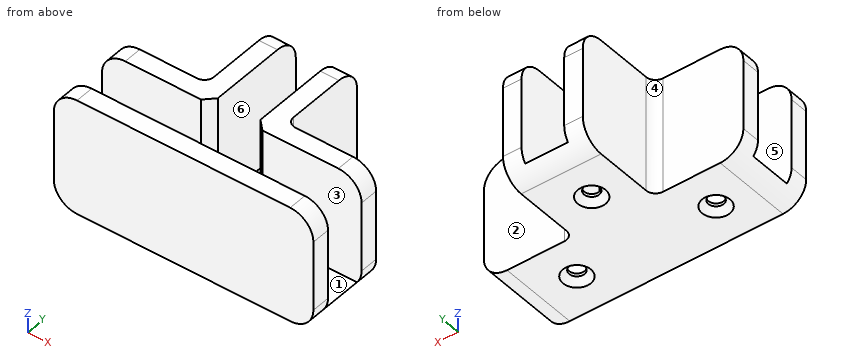
from build123d import *

# Parameters (mm, degrees)
F1_DEPTH       = 2
F2_DEPTH       = 25
F3_R           = 2
F4_T1_DEPTH    = 29
F4_T3_DEPTH    = 29
F4_T5_DEPTH    = 29
F4_T7_DEPTH    = 29
F4_T9_DEPTH    = 42.2
F4_T11_DEPTH   = 42.2
F5_R           = 2
F6_SIZE        = 2
F8_D           = 3.3
F8_CSINK_D     = 6
F8_CSINK_ANGLE = 90


# Not quite as in the source:
# - a fillet or chamfer that OpenCascade refuses, or shapes differently, is made with other operations: its cross-section is extruded or revolved along the edge and cut away or added


with BuildPart() as f1:
    # F0 (on Top) → F1 (new body)
    with BuildSketch(Plane.XY):
        Polygon((-27.6520505063, 0), (0, 0), (28.2951036699, 0), (28.2951036699, 9.2), (4.9215265818, 9.2), (4.9215265818, 32.5735770881), (-4.2784734182, 32.5735770881), (-4.2784734182, 9.2), (-27.6520505063, 9.2), align=None)
        Polygon((28.2951036699, 0), (0, 0), (-27.6520505063, 0), (-27.6520505063, -4), (0, -4), (28.2951036699, -4), align=None)
        Polygon((4.9215265818, 9.2), (28.2951036699, 9.2), (28.2951036699, 13.2), (8.9215265818, 13.2), (8.9215265818, 32.5735770881), (4.9215265818, 32.5735770881), align=None)
        Polygon((-27.6520505063, 13.2), (-27.6520505063, 9.2), (-4.2784734182, 9.2), (-4.2784734182, 32.5735770881), (-8.2784734182, 32.5735770881), (-8.2784734182, 13.2), align=None)
    extrude(amount=F1_DEPTH)

    # F0 (on Top) → F2 (join)
    with BuildSketch(Plane.XY):
        Polygon((-27.6520505063, 13.2), (-27.6520505063, 9.2), (-4.2784734182, 9.2), (-4.2784734182, 32.5735770881), (-8.2784734182, 32.5735770881), (-8.2784734182, 13.2), align=None)
        Polygon((4.9215265818, 9.2), (28.2951036699, 9.2), (28.2951036699, 13.2), (8.9215265818, 13.2), (8.9215265818, 32.5735770881), (4.9215265818, 32.5735770881), align=None)
        Polygon((28.2951036699, 0), (0, 0), (-27.6520505063, 0), (-27.6520505063, -4), (0, -4), (28.2951036699, -4), align=None)
    extrude(amount=F2_DEPTH)

    # F3
    f3_edges = [f1.edges().sort_by_distance(p)[0] for p in [
        (8.921527, 13.2, 12.5),
    ]]
    fillet(f3_edges, radius=F3_R)

    # F4: fillet of radius 5 on 9 edges, made by hand

    # F4_s2 → F4_t1 (cut)
    with BuildSketch(Plane.XZ.offset(-12.5)):
        with BuildLine():
            ThreePointArc((28.2951036699, 20), (26.8306375758, 23.5355339059), (23.2951036699, 25))
            Line((23.2951036699, 25), (28.2951036699, 25))
            Line((28.2951036699, 25), (28.2951036699, 20))
        make_face()
        with BuildLine():
            ThreePointArc((-27.6520505063, 20), (-26.1875844123, 23.5355339059), (-22.6520505063, 25))
            Line((-22.6520505063, 25), (-27.6520505063, 25))
            Line((-27.6520505063, 25), (-27.6520505063, 20))
        make_face()
    extrude(amount=F4_T1_DEPTH, mode=Mode.SUBTRACT)

    # F4_s4 → F4_t3 (cut)
    with BuildSketch(Plane.XZ.offset(-25.7)):
        with BuildLine():
            ThreePointArc((28.2951036699, 20), (26.8306375758, 23.5355339059), (23.2951036699, 25))
            Line((23.2951036699, 25), (28.2951036699, 25))
            Line((28.2951036699, 25), (28.2951036699, 20))
        make_face()
        with BuildLine():
            ThreePointArc((-27.6520505063, 20), (-26.1875844123, 23.5355339059), (-22.6520505063, 25))
            Line((-22.6520505063, 25), (-27.6520505063, 25))
            Line((-27.6520505063, 25), (-27.6520505063, 20))
        make_face()
    extrude(amount=F4_T3_DEPTH, mode=Mode.SUBTRACT)

    # F4_s6 → F4_t5 (cut)
    with BuildSketch(Plane.YZ.offset(-20.7784734182)):
        with BuildLine():
            ThreePointArc((32.5735770881, 20), (31.1091109941, 23.5355339059), (27.5735770881, 25))
            Line((27.5735770881, 25), (32.5735770881, 25))
            Line((32.5735770881, 25), (32.5735770881, 20))
        make_face()
    extrude(amount=F4_T5_DEPTH, mode=Mode.SUBTRACT)

    # F4_s8 → F4_t7 (cut)
    with BuildSketch(Plane.YZ.offset(-7.5784734182)):
        with BuildLine():
            ThreePointArc((32.5735770881, 20), (31.1091109941, 23.5355339059), (27.5735770881, 25))
            Line((27.5735770881, 25), (32.5735770881, 25))
            Line((32.5735770881, 25), (32.5735770881, 20))
        make_face()
    extrude(amount=F4_T7_DEPTH, mode=Mode.SUBTRACT)

    # F4_s10 → F4_t9 (cut)
    with BuildSketch(Plane.XZ.offset(-25.7)):
        with BuildLine():
            ThreePointArc((-22.6520505063, 0), (-26.1875844123, 1.4644660941), (-27.6520505063, 5))
            Line((-27.6520505063, 5), (-27.6520505063, 0))
            Line((-27.6520505063, 0), (-22.6520505063, 0))
        make_face()
        with BuildLine():
            ThreePointArc((23.2951036699, 0), (26.8306375758, 1.4644660941), (28.2951036699, 5))
            Line((28.2951036699, 5), (28.2951036699, 0))
            Line((28.2951036699, 0), (23.2951036699, 0))
        make_face()
    extrude(amount=F4_T9_DEPTH, mode=Mode.SUBTRACT)

    # F4_s12 → F4_t11 (cut)
    with BuildSketch(Plane.YZ.offset(-20.7784734182)):
        with BuildLine():
            ThreePointArc((27.5735770881, 0), (31.1091109941, 1.4644660941), (32.5735770881, 5))
            Line((32.5735770881, 5), (32.5735770881, 0))
            Line((32.5735770881, 0), (27.5735770881, 0))
        make_face()
    extrude(amount=F4_T11_DEPTH, mode=Mode.SUBTRACT)

    # F5
    f5_edges = [f1.edges().sort_by_distance(p)[0] for p in [
        (-8.278473, 13.2, 12.5),
    ]]
    fillet(f5_edges, radius=F5_R)

    # F6
    f6_edges = [f1.edges().sort_by_distance(p)[0] for p in [
        (4.921527, 9.2, 13.5),
        (-4.278473, 9.2, 13.5),
    ]]
    chamfer(f6_edges, length=F6_SIZE)

    # F8 (through all)
    with Locations(Plane(origin=(0, 0, 0), x_dir=(1, 0, 0), z_dir=(0, 0, -1))):
        with Locations((-15, -4.6), (0, -19.6), (15, -4.6)):
            CounterSinkHole(F8_D / 2, F8_CSINK_D / 2, counter_sink_angle=F8_CSINK_ANGLE)


solid = f1.part
Geometry check sheet. Reference: the model listing, model coordinates, mm. Face numbers are marked on the shaded views. A direction names the side the tool comes from. Coordinates: 2 decimals unless noted, no trailing zeros. Write each loop counter-clockwise with the first axis right and the second up, starting at its lowest first coordinate (ties: lowest second). Pieces come first, ordered by that corner, then holes. Notation, with made-up numbers: (-27, 68.5) -> (29, 68.5) arc R11 ccw to (29, 80.5) -> close; hole circle Ø9 at (85, -2). An arc over 180 degrees is marked (long way). One line per question, with ' | ' between items.
1. Cross-section at D-D on x = -15. Record the cut outline in (y, z), and give its area (3 significant figures).
Answers:
outline: (-4, 0) -> (1.6, 0) -> (2.95, 1.35) -> (2.95, 2) -> (0, 2) -> (0, 25) -> (-4, 25) -> close; (6.25, 1.35) -> (7.6, 0) -> (13.2, 0) -> (13.2, 25) -> (9.2, 25) -> (9.2, 2) -> (6.25, 2) -> close | area: 210 mm²
2. Depth check by flat-ended pin: pin 1 Ø12 at (y, z) = (26.5, 18) entering from +X; pin 2 Ø3 at (y, z) = (23.5, 14.5) entering from -X; pin 3 Ø5 at (x, z) = (22.5, 9) entering from +Y; pin 4 Ø2 at (x, y) = (15, 4.6) entering from -Z. Enter the tip coordinate at first touch or a pass-through.
Answers:
pin 1: stops at x = 8.92 | pin 2: stops at x = -8.28 | pin 3: stops at y = 13.2 | pin 4: passes through
3. Cross-section at A-A on x = 0. Record the cut outline in (y, z).
Answers:
outline: (-4, 0) -> (16.6, 0) -> (17.95, 1.35) -> (17.95, 2) -> (0, 2) -> (0, 25) -> (-4, 25) -> close; (21.25, 1.35) -> (22.6, 0) -> (27.57, 0) arc R5 ccw to (31.57, 2) -> (21.25, 2) -> close
4. Set-up check for the marked faces 1, 2 and 3: record each of +Z, -Z, +X, -X, +Y, -Y from which the full face is reachable in a straight line by a thin tool's end or side.
Answers:
face 1: +Z | face 2: +Z, -Z, +X, +Y | face 3: +Z, +X, -X
5. Cross-section at B-B on y = 19.6. Record the cut outline in (x, z), and give its area (3 significant figures).
Answers:
outline: (-8.28, 0) -> (-3, 0) -> (-1.65, 1.35) -> (-1.65, 2) -> (-4.28, 2) -> (-4.28, 25) -> (-8.28, 25) -> close; (1.65, 1.35) -> (3, 0) -> (8.92, 0) -> (8.92, 25) -> (4.92, 25) -> (4.92, 2) -> (1.65, 2) -> close | area: 210 mm²
6. Draft check along Y on the marked faces 4, 5 and 6. Enter one of: +Y half, -Y half, draft (parallel to the pull), parting line (faces both ways), or undercut.
Answers:
face 4: +Y half | face 5: undercut | face 6: draft
7. Cross-section at C-C on y = 4.6. Record the cut outline in (x, z).
Answers:
outline: (-26.65, 2) arc R5 ccw to (-22.65, 0) -> (-18, 0) -> (-16.65, 1.35) -> (-16.65, 2) -> close; (-13.35, 1.35) -> (-12, 0) -> (12, 0) -> (13.35, 1.35) -> (13.35, 2) -> (-13.35, 2) -> close; (16.65, 1.35) -> (18, 0) -> (23.3, 0) arc R5 ccw to (27.3, 2) -> (16.65, 2) -> close
8. Thickness scan on probe 1 along X at (y, z) = (16, 11); probe 2 along Y at (x, z) = (-22, 2.25); probe 3 along X at (y, z) = (4.6, 1.65). Record the ranges inside material, lowest first. Write a range as from..to.
Answers:
probe 1: x = -8.28..-4.28, 4.92..8.92 | probe 2: y = -4..0, 9.2..13.2 | probe 3: x = -26.36..-16.65, -13.35..13.35, 16.65..27.01
